Source: CAD feature listing. Evaluate the final solid. Frame: model axes, mm. A direction names the side the tool comes from. Round coordinates to 2 decimals unless told otherwise and drop trailing zeros. Loops run counter-clockwise (first coordinate to the right, second up) from the corner with the lowest first, then second, coordinate; pieces in that order, holes last. Notation, with made-up numbers: (49.5, 71) -> (90.5, 71) arc R21 ccw to (90.5, 85) -> close; hole circle Ø9 at (8, 27.25). An arc over 180 degrees is marked (long way). Write item = value, one per line.
from build123d import *

# Parameters (mm, degrees)
F0_R         = 5
F1_DEPTH     = 6
F3_R         = 15
F4_DEPTH     = 25
F5_R         = 3.75
F6_DEPTH     = 10
F8_DEPTH     = 2
F9_DEPTH     = 2
F10_T1_DEPTH = 55.6511992514
F11_T1_DEPTH = 55.6511992514
F12_SIZE2    = 23
F12_SIZE     = 10
F14_W        = 12
F14_H        = 12
F15_DEPTH    = 1
F16_W        = 12
F16_H        = 12
F17_DEPTH    = 1
F18_SIZE2    = 7
F18_SIZE     = 2
F19_SIZE2    = 7
F19_SIZE     = 2


# Not quite as in the source:
# - a fillet or chamfer that OpenCascade refuses, or shapes differently, is made with other operations: its cross-section is extruded or revolved along the edge and cut away or added
# - two fillets or chamfers of one size are made in one step


with BuildPart() as f1:
    # F0 (on Top) → F1 (new body)
    with BuildSketch(Plane.XY):
        Circle(F0_R)
    extrude(amount=F1_DEPTH)

    # F3 (on offset) → F4 (cut)
    with BuildSketch(Plane.XZ.offset(6)):
        with Locations((0, -14)):
            Circle(F3_R)
    extrude(amount=-F4_DEPTH, mode=Mode.SUBTRACT)

    # F5 (on face) → F6 (join)
    with BuildSketch(Plane.XY.offset(6)):
        Circle(F5_R)
    extrude(amount=-F6_DEPTH)

    # F7 (on Right) → F8 (join)
    with BuildSketch(Plane.YZ):
        Polygon((16, 3), (16, 37), (-16, 37), (-16, 3), (0, 3), align=None)
    extrude(amount=F8_DEPTH)

    # F9 (add): a face of the model
    f9_faces = [f1.faces().sort_by_distance(p)[0] for p in [
        (0, 0, 20.4395085066),
    ]]
    extrude(f9_faces, amount=F9_DEPTH)

    # F10: chamfer of 10 x 7 on 1 edges, made by hand

    # F10_s2 → F10_t1 (cut)
    with BuildSketch(Plane.YZ.offset(-27.8255996257)):
        Polygon((-16, 10), (-6, 3), (-16, 3), align=None)
    extrude(amount=F10_T1_DEPTH, mode=Mode.SUBTRACT)

    # F11: chamfer of 7 x 10 on 1 edges, made by hand

    # F11_s2 → F11_t1 (cut)
    with BuildSketch(Plane.YZ.offset(-27.8255996257)):
        Polygon((6, 3), (16, 10), (16, 3), align=None)
    extrude(amount=F11_T1_DEPTH, mode=Mode.SUBTRACT)

    # F12
    f12_edges = [f1.edges().sort_by_distance(p)[0] for p in [
        (0, -16, 37),
        (0, 16, 37),
    ]]
    f12_side = f1.faces().sort_by_distance((0, 0, 37))[0]
    chamfer(f12_edges, length=F12_SIZE, length2=F12_SIZE2, reference=f12_side)

    # F14 (on face) → F15 (join)
    with BuildSketch(Plane(origin=(-2, 0, 0), x_dir=(0, -1, 0), z_dir=(-1, 0, 0))):
        with Locations((0, 9)):
            Rectangle(F14_W, F14_H)
    extrude(amount=F15_DEPTH)

    # F16 (on face) → F17 (join)
    with BuildSketch(Plane.YZ.offset(2)):
        with Locations((0, 9)):
            Rectangle(F16_W, F16_H)
    extrude(amount=F17_DEPTH)

    # F18
    f18_edges = [f1.edges().sort_by_distance(p)[0] for p in [
        (-2.5, -6, 15),
        (-2.5, 6, 15),
    ]]
    f18_side = f1.faces().sort_by_distance((-2.5, 0, 15))[0]
    chamfer(f18_edges, length=F18_SIZE, length2=F18_SIZE2, reference=f18_side)

    # F19
    f19_edges = [f1.edges().sort_by_distance(p)[0] for p in [
        (2.5, 6, 15),
        (2.5, -6, 15),
    ]]
    f19_side = f1.faces().sort_by_distance((2.5, 0, 15))[0]
    chamfer(f19_edges, length=F19_SIZE, length2=F19_SIZE2, reference=f19_side)


solid = f1.part
1. Mould query, pull axis Y, two halves, no side actions, for faces 6 (the face through (2.5, -6, 5.5)), 7 (the face through (-2.5, 5, 11.5)), 8 (the face through (0, 5.4, 3)). Classes: released by +Y, released by -Y, zero draft, split by the parting line, or undercut.
Evaluation:
face_6 = released by -Y
face_7 = released by +Y
face_8 = zero draft
2. Section query B-B (x = -1.25). Return the cut outline in (y, z).
Evaluation:
outline = (-16, 10) -> (-6, 3) -> (-5, 3) -> (-5, 6) -> (-4.84, 6) -> (-4.84, 0.95) -> (-3.54, 0.95) -> (-3.54, -4) -> (3.54, -4) -> (3.54, 0.95) -> (4.84, 0.95) -> (4.84, 6) -> (5, 6) -> (5, 3) -> (6, 3) -> (16, 10) -> (16, 14) -> (6, 37) -> (-6, 37) -> (-16, 14) -> close
3. Section query C-C (y = 14). Return the cut outline in (x, z).
Evaluation:
outline = (-2, 8.6) -> (2, 8.6) -> (2, 18.6) -> (-2, 18.6) -> close
4. Section query D-D (z = 7). Return the cut outline in (x, y).
Evaluation:
outline = (-3, -6) -> (-2, -6) -> (-2, -11.71) -> (2, -11.71) -> (2, -6) -> (3, -6) -> (3, 6) -> (2, 6) -> (2, 11.71) -> (-2, 11.71) -> (-2, 6) -> (-3, 6) -> close
5. Set-up query: faces 1 (the face through (3.464, -1.436, -1.464)), 2 (the face through (4, 0, 6)), 3 (the face through (-2.5, -5, 11.5)), 4 (the face through (2.5, -5, 11.5)), 5 (the face through (-2.5, 6, 5.5)). Return all of +Z, -Z, +X, -X, +Y, -Y with unobstructed straight access to the full face (end or side cutting, diameter ignored); none if empty.
Evaluation:
face_1 = -Z
face_2 = +Z, +X, +Y, -Y
face_3 = +Z, -X, -Y
face_4 = +Z, +X, -Y
face_5 = +Z, -Z, -X, +Y
6. Contact query for flat-ended pins moving along their axis: pin 1 Ø9.5 at (y, z) = (-2, 15.5) entering from -X; pin 2 Ø12 at (y, z) = (-3.5, 7.5) entering from -X; pin 3 Ø1.6 at (x, z) = (-1, 5) entering from -Y; pin 4 Ø0.8 at (x, y) = (-2.5, -2) entering from +Z. Output: stop coordinate, or through.
Evaluation:
pin_1 = -3
pin_2 = -5
pin_3 = -10
pin_4 = 15
7. Section query A-A (z = 12). Return the cut outline in (x, y), then the cut area to 3 significant figures.
Evaluation:
outline = (-3, -4.86) -> (-2, -4.86) -> (-2, -16) -> (2, -16) -> (2, -4.86) -> (3, -4.86) -> (3, 4.86) -> (2, 4.86) -> (2, 16) -> (-2, 16) -> (-2, 4.86) -> (-3, 4.86) -> close
area = 147 mm²
8. Line query: probe 1 along Z at (x, y) = (2.75, -1); probe 2 along X at (y, z) = (-14, 16.5); probe 3 along Y at (x, z) = (-4, 0.5). Output: solid intervals per line, ascending. Write a range as from..to.
Evaluation:
probe_1 = -4..15
probe_2 = -2..2
probe_3 = -3..3
